Can you work these out from the model? Positions are in its coordinate system, mm. A direction names the side the tool comes from. Coordinates: 2 decimals unless noted, no trailing zeros. Order: outer loops, then holes, each group sorted by start corner. A loop starts at its lowest first (then second) coordinate and runs counter-clockwise, first axis right, second up. Notation, with made-up numbers: (74, 42) -> (128, 42) arc R6 ccw to (128, 52) -> close; hole circle Ø6 at (1, -38). An arc over 180 degrees is marked (long way). Return JSON: item names as keys, results as strings. Group by question number.
1) If we section it at B-B, the plane y = 0: Please give me the cut outline in (x, z), then the cut area to 3 significant figures.
2) For pin 1 (5 mm diameter, centred on y = 0, z = 6.5, fed in from -X); pin 2 (2 mm diameter, centred on x = -4.5, z = 10, fed in from +Y); pin 3 (3 mm diameter, centred on y = -5, z = 47, fed in from -X); pin 4 (5 mm diameter, centred on x = 4.5, y = -4.5, fed in from +Z), each with a flat end and sliding along its axis, tell me the tip position at first contact or that it passes through.
3) If we section it at A-A, the plane x = 0: Please give me the cut outline in (y, z).
4) If I drill on probe 1 along Z at (x, y) = (-1, 0); probe 2 along Y at (x, z) = (0.25, 6.5); probe 3 along Y at (x, z) = (5.75, 58.5), over which ranges is the centre line in solid material (lowest first)? Write a range as from..to.
5) For faces 4 (the cylindrical face through (6.466, -2.681, 29.583)), 5 (the flat face through (6, 0, 60)), which set-ups out of +Z, -Z, +X, -X, +Y, -Y let a thin tool reach every point of the face, with its end or its side?
6) If we section it at D-D, the plane z = 6.5: Please give me the cut outline in (x, y).
7) Thinking about a two-plate mould opening in Y: for faces 1 (the cylindrical face through (-1.19, -5.37, 61.38)), 2 (the cylindrical face through (-0.1, 2.7, 9.45)), 3 (the flat face through (0, 0, 63)), which applies, +Y half, -Y half, draft (parallel to the pull), parting line (faces both ways), or undercut?
8) If we section it at C-C, the plane z = 20: Please give me the cut outline in (x, y), then the cut area to 3 significant figures.
from build123d import *

# Parameters (mm, degrees)
SKIZZE1_R                            = 7
AUFSATZ_LINEAR_AUSTRAGEN1_DEPTH      = 60
SKIZZE2_R                            = 5.5
AUFSATZ_LINEAR_AUSTRAGEN2_DEPTH      = 3
SCHNITT_LINEAR_AUSTRAGEN2_DEPTH      = 64.773035054
SCHNITT_LINEAR_AUSTRAGEN2_DEPTH_BACK = 64.773035054
SKIZZE4_R                            = 4
FASE1_SIZE                           = 0.2


with BuildPart() as part:
    # Skizze1 → Aufsatz-Linear austragen1 (new body)
    with BuildSketch(Plane.XY):
        Circle(SKIZZE1_R)
    extrude(amount=AUFSATZ_LINEAR_AUSTRAGEN1_DEPTH)

    # Skizze2 → Aufsatz-Linear austragen2 (add)
    with BuildSketch(Plane.XY.offset(60)):
        Circle(SKIZZE2_R)
    extrude(amount=AUFSATZ_LINEAR_AUSTRAGEN2_DEPTH)

    # Skizze4 → Schnitt-Linear austragen2 (cut, two sides: drawn at the far end of the back side and taken through both)
    with BuildSketch(Plane(origin=(0, 0, 0), x_dir=(0, 0, -1), z_dir=(1, 0, 0)).offset(-SCHNITT_LINEAR_AUSTRAGEN2_DEPTH_BACK)):
        with Locations((-6.5, 0)):
            Circle(SKIZZE4_R)
    extrude(amount=SCHNITT_LINEAR_AUSTRAGEN2_DEPTH + SCHNITT_LINEAR_AUSTRAGEN2_DEPTH_BACK, mode=Mode.SUBTRACT)

    # Fase1
    fase1_edges = [part.edges().sort_by_distance(p)[0] for p in [
        (-7, 0, 0),
        (-7, 0, 60),
        (-5.5, 0, 63),
    ]]
    chamfer(fase1_edges, length=FASE1_SIZE)


solid = part.part
Result sheet:
{
 "1": {"outline": "(-7, 0.2) -> (-6.8, 0) -> (6.8, 0) -> (7, 0.2) -> (7, 2.5) -> (-7, 2.5) -> close; (-7, 10.5) -> (7, 10.5) -> (7, 59.8) -> (6.8, 60) -> (5.5, 60) -> (5.5, 62.8) -> (5.3, 63) -> (-5.3, 63) -> (-5.5, 62.8) -> (-5.5, 60) -> (-6.8, 60) -> (-7, 59.8) -> close", "area": "761 mm2"},
 "2": {"pin 1": "passes through", "pin 2": "stops at y = 6.06", "pin 3": "stops at x = -6.06", "pin 4": "stops at z = 63"},
 "3": {"outline": "(-7, 0.2) -> (-6.8, 0) -> (6.8, 0) -> (7, 0.2) -> (7, 59.8) -> (6.8, 60) -> (5.5, 60) -> (5.5, 62.8) -> (5.3, 63) -> (-5.3, 63) -> (-5.5, 62.8) -> (-5.5, 60) -> (-6.8, 60) -> (-7, 59.8) -> close; hole circle Ø8 at (0, 6.5)"},
 "4": {"probe 1": "z = 0..2.5, 10.5..63", "probe 2": "y = -7..-4, 4..7", "probe 3": "y = -3.99..3.99"},
 "5": {"face 4": "+Z, -Z", "face 5": "+Z"},
 "6": {"outline": "(-5.74, -4) arc R7 ccw to (5.74, -4) -> close; (-5.74, 4) -> (5.74, 4) arc R7 ccw to start"},
 "7": {"face 1": "parting line", "face 2": "undercut", "face 3": "draft"},
 "8": {"outline": "circle Ø14 at (0, 0)", "area": "154 mm2"}
}
